The figure shows three views and two pictorial views of one solid part (mm, origin at its lowest corner). Answer the questions. A direction names the side the tool comes from. Coordinates: 2 decimals unless noted, no trailing zeros. Order: outer loops, then holes, each group sorted by start corner. A loop starts at its lowest first (then second) coordinate and runs counter-clockwise, first axis right, second up. Notation, with made-up numbers: (85.25, -25.75) -> (93.25, -25.75) arc R20 cw to (93.25, -17.75) -> close; hole circle Ø7 at (-0.5, 70). An arc over 180 degrees is marked (long way). Return JSON: item names as keys, results as strings. Group by question number.
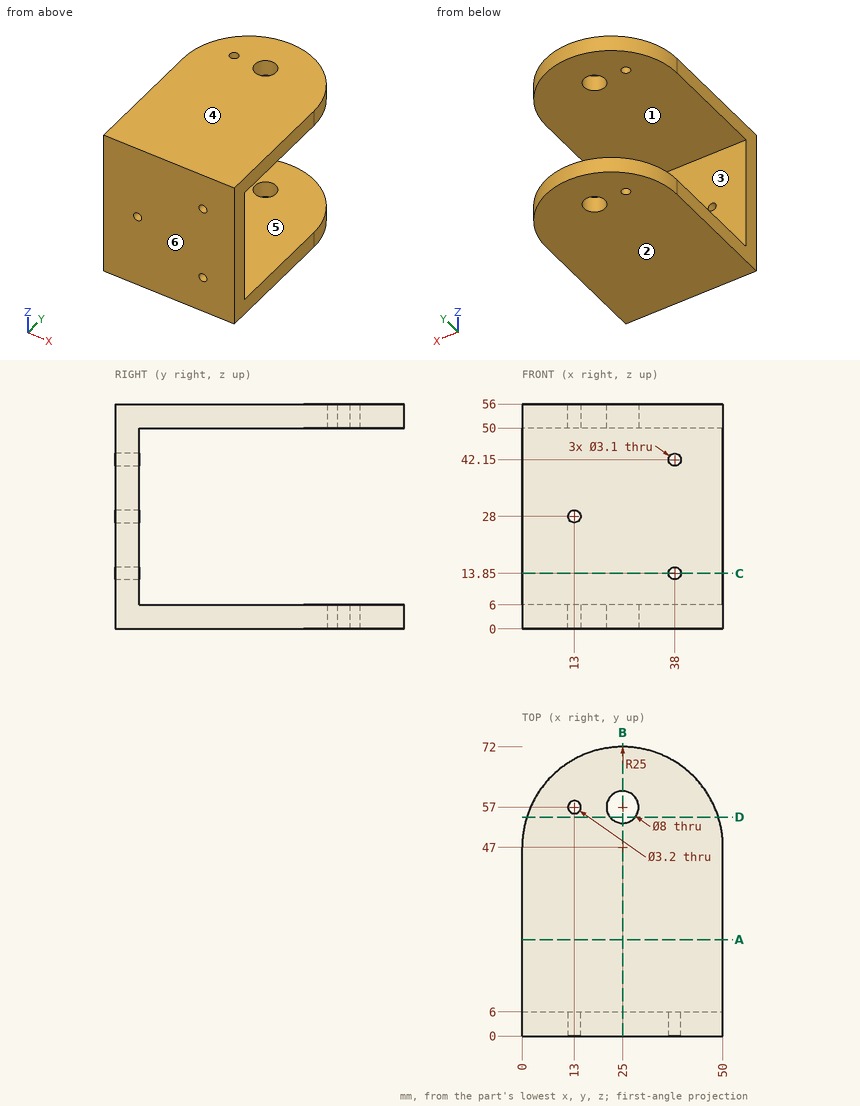
1. Find section C-C on z = 13.85. Determine the outline of the cut face in (x, y), and give its area (3 significant figures).
2. Given pin 1 (6.5 mm diameter, centred on x = 25, y = 57, fed in from -Z); pin 2 (1 mm diameter, centred on x = 9, z = 12.5, fed in from +Y); pin 3 (12 mm diameter, centred on x = 15.5, z = 48.5, fed in from +Y), each flat-ended and moving along its own axis, determine where each tip first touches the part or whether it passes through.
3. Find section B-B on x = 25. Determine the outline of the cut face in (y, z).
4. Straight lines are drawn through the part: L1, parallel to Z at x = 25.5, y = 66; L2, parallel to Y at x = 25, z = 1; L3, parallel to Y at x = 42.5, z = 25. For each, find the intervals that lie inside material, in ascending order.
5. Find section A-A on y = 24. Determine the outline of the cut face in (x, z).
6. Which of the six approach directions +Z, -Z, +X, -X, +Y, -Y give full straight-line access (tool end or side, diameter ignored) to the marked faces 1 and 2?
7. For a pull along Z with two mould halves and no side action, classify the marked faces 3, 4, 5 and 6 as released by +Z, released by -Z, zero draft, split by the parting line, or undercut.
8. Find section D-D on y = 54.5. Determine the outline of the cut face in (x, z).
Result:
{
 "1": {"outline": "(0, 0) -> (36.45, 0) -> (36.45, 6) -> (0, 6) -> close; (39.55, 0) -> (50, 0) -> (50, 6) -> (39.55, 6) -> close", "area": "281 mm^2"},
 "2": {"pin 1": "through", "pin 2": "y = 6", "pin 3": "y = 71.73"},
 "3": {"outline": "(0, 0) -> (53, 0) -> (53, 6) -> (6, 6) -> (6, 50) -> (53, 50) -> (53, 56) -> (0, 56) -> close; (61, 0) -> (72, 0) -> (72, 6) -> (61, 6) -> close; (61, 50) -> (72, 50) -> (72, 56) -> (61, 56) -> close"},
 "4": {"L1": "0 to 6, 50 to 56", "L2": "0 to 53, 61 to 72", "L3": "0 to 6"},
 "5": {"outline": "(0, 0) -> (50, 0) -> (50, 6) -> (0, 6) -> close; (0, 50) -> (50, 50) -> (50, 56) -> (0, 56) -> close"},
 "6": {"face 1": "+X, -X, +Y", "face 2": "-Z, +X, -X, +Y, -Y"},
 "7": {"face 3": "undercut", "face 4": "released by +Z", "face 5": "undercut", "face 6": "zero draft"},
 "8": {"outline": "(1.15, 0) -> (21.88, 0) -> (21.88, 6) -> (1.15, 6) -> close; (1.15, 50) -> (21.88, 50) -> (21.88, 56) -> (1.15, 56) -> close; (28.12, 0) -> (48.85, 0) -> (48.85, 6) -> (28.12, 6) -> close; (28.12, 50) -> (48.85, 50) -> (48.85, 56) -> (28.12, 56) -> close"}
}
